```python
from build123d import *

# Parameters (mm, degrees)
F0_R     = 12.9
F1_DEPTH = 15
F2_T     = -1.4
F3_R     = 6


with BuildPart() as f1:
    # F0 (on Top) → F1 (new body)
    with BuildSketch(Plane.XY):
        Circle(F0_R)
    extrude(amount=F1_DEPTH)

    # F2
    f2_openings = [f1.faces().sort_by_distance(p)[0] for p in [
        (0, 0, 15),
    ]]
    offset(amount=F2_T, openings=f2_openings)

    # F3
    f3_edges = [f1.edges().sort_by_distance(p)[0] for p in [
        (-11.5, 0, 1.4),
        (-12.9, 0, 0),
    ]]
    fillet(f3_edges, radius=F3_R)


solid = f1.part
```
The model under review builds one solid part; all positions refer to its coordinate system, in mm. Give positions to 0.01 mm unless a question says otherwise; leave off trailing zeros. Loops run counter-clockwise (first coordinate to the right, second up) from the corner with the lowest first, then second, coordinate; pieces in that order, holes last. Notation, with made-up numbers: (-18.75, 7) - (-1.75, 7) arc R25 cw to (-1.75, 44) - close; hole circle Ø7 at (51, 22). An arc over 180 degrees is marked (long way). Answer as a JSON object with one key per item and string values.
Q1. Add section A-A on z = 14.25. State the section outline as (x, y) points.
Worked out:
{"outline": "circle Ø25.8 at (0, 0); hole circle Ø23 at (0, 0)"}
Q2. Insertion check: pin 1 (9 mm diameter, centred on x = -1.5, y = -0.5, fed in from +Z); pin 2 (3 mm diameter, centred on y = 4, z = 11.5, fed in from +X); pin 3 (8 mm diameter, centred on x = -4.5, y = -8, fed in from +Z); pin 4 (1.5 mm diameter, centred on y = 10.5, z = 2.5, fed in from +X). Each pin has a flat end and moves straight along its axis. Give the tip position at first contact, or say it passes through.
Worked out:
{"pin 1": "stops at z = 1.43", "pin 2": "stops at x = 12.66", "pin 3": "stops at z = 15", "pin 4": "stops at x = 6.9"}
Q3. To check wall thickness, follow line 1 along Y through (x, z) = (0, 11.75); line 2 along X through (y, z) = (5.25, 13); line 3 along Y through (x, z) = (-4, 10.5). State the ranges of each line that lie inside material, in increasing order.
Worked out:
{"line 1": "y = -12.9 to -11.5, 11.5 to 12.9", "line 2": "x = -11.78 to -10.23, 10.23 to 11.78", "line 3": "y = -12.26 to -10.78, 10.78 to 12.26"}
Q4. Mouldability with a two-part tool opening along X and no side actions: class faces 1 (the cylindrical face through (-1.5, 11.4, 11.1)), 2 (the flat face through (0, 0, 1.4)), 3 (the flat face through (-9, -8, 15)), 4 (the cylindrical face through (-2.796, -12.593, 10.437)) as +X half, -X half, draft (parallel to the pull), parting line (faces both ways), or undercut.
Worked out:
{"face 1": "undercut", "face 2": "undercut", "face 3": "draft", "face 4": "parting line"}
